Here's the drawing with two shaded views (mm, measured from the low corner). I have some questions. A direction names the side the tool comes from. Coordinates: 2 decimals unless noted, no trailing zeros. Loops run counter-clockwise (first coordinate to the right, second up) from the corner with the lowest first, then second, coordinate; pieces in that order, holes last.
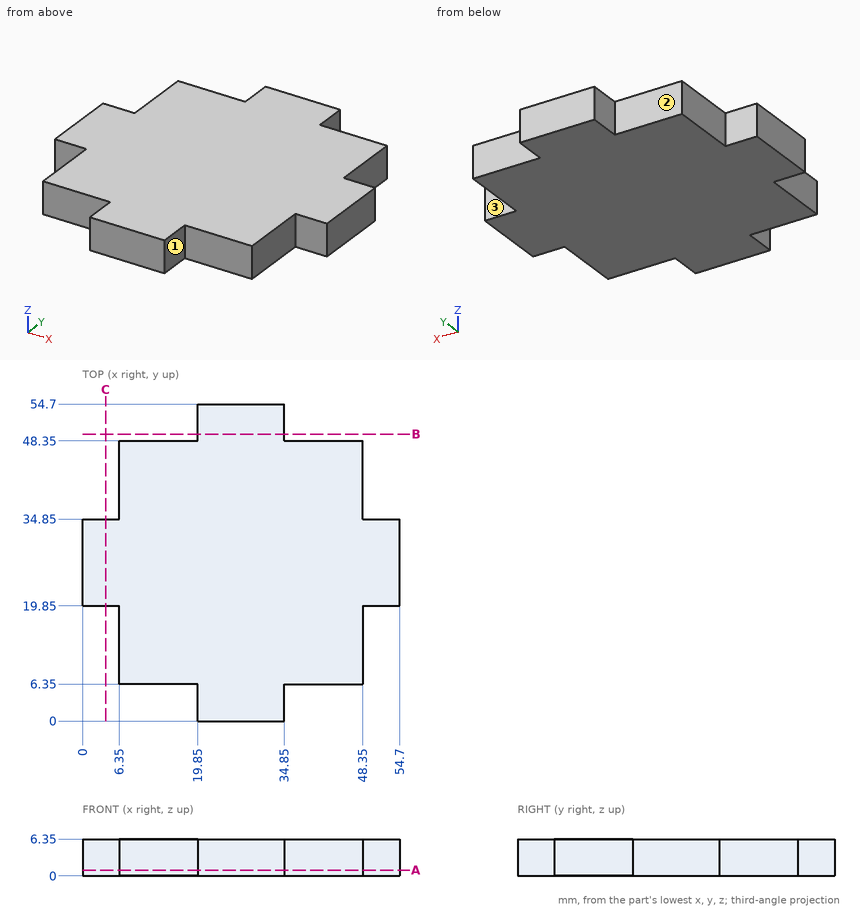
Q1. For the marked faces 1, 2 and 3, which set-ups out of +Z, -Z, +X, -X, +Y, -Y let a thin tool reach every point of the face, with its end or its side?
Q2. Suppose I cut it at B-B on y = 49.5. Write out the boundary of the cut face in (x, z).
Q3. Please list where these lines run through material, in increasing order: probe 1 along X at (y, z) = (8.5, 3.75); probe 2 along X at (y, z) = (51.5, 4.75).
Q4. Will these pins go through, and if not, where does the flat tip stop? P1, Ø3, axis at y = 37, z = 2, coming from the +X side; P2, Ø1.9, axis at y = 4, z = 3, coming from the +X side; P3, Ø1.9, axis at y = 4, z = 4, coming from the -X side.
Q5. Suppose I cut it at A-A on z = 1. Write out the boundary of the cut face in (x, y).
Check values:
1. face 1: +Z, -Z, +X, -Y
1. face 2: +Z, -Z, -X, +Y
1. face 3: +Z, -Z, +X, +Y
2. outline: (19.85, 0) - (34.85, 0) - (34.85, 6.35) - (19.85, 6.35) - close
3. probe 1: x = 6.35 to 48.35
3. probe 2: x = 19.85 to 34.85
4. P1: stops at x = 48.35
4. P2: stops at x = 34.85
4. P3: stops at x = 19.85
5. outline: (0, 19.85) - (6.35, 19.85) - (6.35, 6.35) - (19.85, 6.35) - (19.85, 0) - (34.85, 0) - (34.85, 6.35) - (48.35, 6.35) - (48.35, 19.85) - (54.7, 19.85) - (54.7, 34.85) - (48.35, 34.85) - (48.35, 48.35) - (34.85, 48.35) - (34.85, 54.7) - (19.85, 54.7) - (19.85, 48.35) - (6.35, 48.35) - (6.35, 34.85) - (0, 34.85) - close
